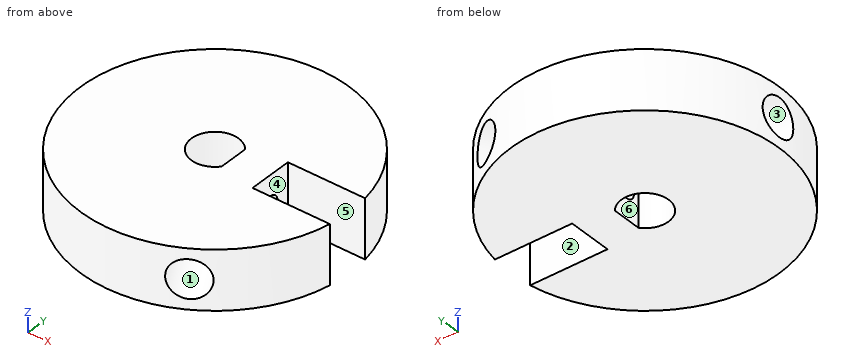
from build123d import *

# Parameters (mm, degrees)
F1_DEPTH = 8
F2_R     = 1.25
F3_DEPTH = 5
F5_R     = 2.6
F6_DEPTH = 25
F7_COUNT = 3
F7_ANGLE = 240


with BuildPart() as f1:
    # F0 (on Top) → F1 (new body)
    with BuildSketch(Plane.XY):
        with BuildLine():
            Line((7.5, 3), (18.001736, 3))
            ThreePointArc((18.001736, 3), (-18.25, 0), (18.001736, -3))
            Line((18.001736, -3), (7.5, -3))
            Line((7.5, -3), (7.5, 0))
            Line((7.5, 0), (7.5, 3))
        make_face()
        with BuildLine():
            ThreePointArc((2.5, -1.997498), (-3.2, 0), (2.5, 1.997498))
            Line((2.5, 1.997498), (2.5, -1.997498))
        make_face(mode=Mode.SUBTRACT)
    extrude(amount=F1_DEPTH)

    # F2 (on face) → F3 (cut, through all)
    with BuildSketch(Plane.YZ.offset(7.5)):
        with Locations((0, 4)):
            Circle(F2_R)
    extrude(amount=-F3_DEPTH, mode=Mode.SUBTRACT)


with BuildPart() as f6:
    # F5 (on offset) → F6 (new body)
    with BuildSketch(Plane.YZ.offset(-10)):
        with Locations((0, 4)):
            Circle(F5_R)
    extrude(amount=-F6_DEPTH)


with BuildPart() as f7_1:
    # F7: instance of F6
    add(f6.part.rotate(Axis((0, 0, 0), (0, 0, -1)), 1 * F7_ANGLE / (F7_COUNT - 1)))


with BuildPart() as f7_2:
    # F7: instance of F6
    add(f6.part.rotate(Axis((0, 0, 0), (0, 0, -1)), 2 * F7_ANGLE / (F7_COUNT - 1)))


with BuildPart() as f1_1:
    add(f1.part)

    # F8: cut F6, F7_1, F7_2
    add(f6.part, mode=Mode.SUBTRACT)
    add(f7_1.part, mode=Mode.SUBTRACT)
    add(f7_2.part, mode=Mode.SUBTRACT)


solid = f1_1.part
Part model, mm, in its own coordinate system. Face numbers are marked on the shaded views. A direction names the side the tool comes from. Coordinates: 2 decimals unless noted, no trailing zeros. Loops run counter-clockwise (first coordinate to the right, second up) from the corner with the lowest first, then second, coordinate; pieces in that order, holes last. Notation, with made-up numbers: M -19,55.5 L 20,55.5 A25 cw 20,75.5 Z; hole C -37,-20 d4. An arc over 180 degrees is marked long. Use a Markdown table: item, result. Add a question column.
Q1. Mould opens along X. For the marked faces 4, 5 and 6 say: +X half, -X half, draft (parallel to the pull), parting line (faces both ways), or undercut.
Q2. Probe L1, parallel to Z at x = -14.25, y = 0; L2, parallel to Y at x = 5, z = 5; L3, parallel to Y at x = 4, z = 6. List the from-to ranges inside material, lowest first.
Q3. Cut at D-D (z = 4.5). Write the cut outline in (x, y), and give its area (3 significant figures).
Q4. Cut at A-A (y = 0). Write the cut outline in (x, z), and give its area (3 significant figures).
Q5. Cut at C-C (z = 2.25). Write the cut outline in (x, y).
Q6. Cut at B-B (x = 0). Write the cut outline in (y, z), and give its area (3 significant figures).
Q7. Pin check, flat tips, straight feed: P1, Ø4, axis at x = 11.5, z = 5, coming from the +Y side; P2, Ø4, axis at x = 13.5, z = 3.5, coming from the -Y side; P3, Ø4, axis at y = 0.5, z = 3.5, coming from the -X side. Stop position of each tip, or through.
Q8. Which spindle directions (+Z, -Z, +X, -X, +Y, -Y) get a long thin tool onto all of the face, cutting with end or side? Do the marked faces 1, 2 and 3. Say none if no direction does.
Worked out:
| question | item | result |
|---|---|---|
| 1 | face 4 | +X half |
| 1 | face 5 | draft |
| 1 | face 6 | undercut |
| 2 | L1 | z = 0 to 1.4, 6.6 to 8 |
| 2 | L2 | y = -17.55 to -13.46, -8.66 to -0.75, 0.75 to 8.66, 13.46 to 17.55 |
| 2 | L3 | y = -17.81 to -10.25, -9.24 to 9.24, 10.25 to 17.81 |
| 3 | outline | M -18.07,-2.55 A18.25 ccw 6.83,-16.93 L 2.79,-9.94 L 7.21,-7.38 L 11.25,-14.37 A18.25 ccw 18,-3 L 7.5,-3 L 7.5,-1.15 L 2.5,-1.15 L 2.5,-2 A3.2 cw long 2.5,2 L 2.5,1.15 L 7.5,1.15 L 7.5,3 L 18,3 A18.25 ccw 11.25,14.37 L 7.21,7.38 L 2.79,9.94 L 6.83,16.93 A18.25 ccw -18.07,2.55 L -10,2.55 L -10,-2.55 Z |
| 3 | area | 815 mm2 |
| 4 | outline | M -18.25,0 L -3.2,0 L -3.2,8 L -18.25,8 L -18.25,6.6 L -10,6.6 L -10,1.4 L -18.25,1.4 Z; M 2.5,0 L 7.5,0 L 7.5,2.75 L 2.5,2.75 Z; M 2.5,5.25 L 7.5,5.25 L 7.5,8 L 2.5,8 Z |
| 4 | area | 105 mm2 |
| 5 | outline | M -18.15,-1.92 A18.25 ccw 7.41,-16.68 L 3.33,-9.62 L 6.67,-7.7 L 10.74,-14.76 A18.25 ccw 18,-3 L 7.5,-3 L 7.5,3 L 18,3 A18.25 ccw 10.74,14.76 L 6.67,7.7 L 3.33,9.62 L 7.41,16.68 A18.25 ccw -18.15,1.92 L -10,1.92 L -10,-1.92 Z; hole M 2.5,-2 L 2.5,2 A3.2 ccw long Z |
| 6 | outline | M -18.25,0 L -3.2,0 L -3.2,8 L -18.25,8 Z; M 3.2,0 L 18.25,0 L 18.25,8 L 3.2,8 Z |
| 6 | area | 241 mm2 |
| 7 | P1 | stops at y = 15.24 |
| 7 | P2 | stops at y = -14.17 |
| 7 | P3 | stops at x = -18.23 |
| 8 | face 1 | none |
| 8 | face 2 | +Z, -Z, +X |
| 8 | face 3 | -X |
